Build history of the part. All positions in model axes, mm. Round coordinates to 2 decimals unless told otherwise and drop trailing zeros. Order: outer loops, then holes, each group sorted by start corner. A loop starts at its lowest first (then second) coordinate and runs counter-clockwise, first axis right, second up. Notation, with made-up numbers: M 1,53 L 52,53 A26 ccw 52,91 Z; hole C 41,51 d6. An arc over 180 degrees is marked long. One line per item, written item: value. Start each with the question number.
Item 1: Band-saw the part on A-A, the plane z = 262. Write the cut outline in (x, y).
Item 2: Band-saw the part on B-B, the plane z = 329. Write the cut outline in (x, y), then the cut area to 3 significant figures.
Item 3: Pin check, flat tips, straight feed: pin 1 (2 mm diameter, centred on y = 20, z = 311.5, fed in from -X); pin 2 (4 mm diameter, centred on y = 50.8, z = 101.6, fed in from -X); pin 3 (0.8 mm diameter, centred on x = 0.5, y = 27, fed in from -Z). Stop position of each tip, or through.
Item 4: Probe L1, parallel to Z at x = 0.4, y = 6.35; L2, parallel to Y at x = 0.55, z = 139.7; L3, parallel to Z at x = 0.1, y = -13. List the from-to ranges inside material, lowest first.
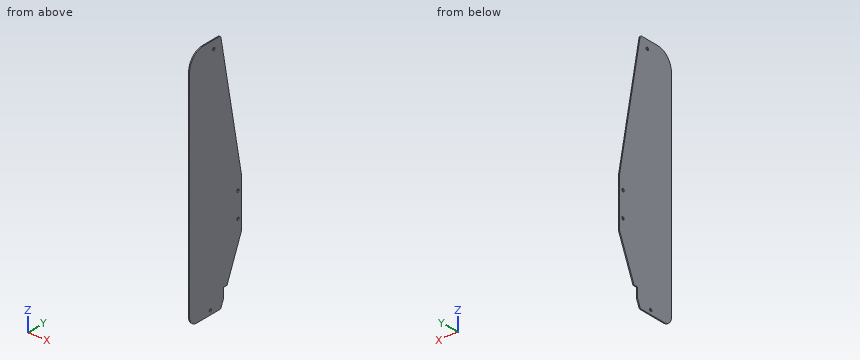
Autodesk Inventor part; units mm, degrees
ref_plane "YZ Plane" through (0, 0, 0) normal (1, 0, 0) x (0, 1, 0)
ref_plane "XZ Plane" through (0, 0, 0) normal (0, 1, 0) x (-1, 0, 0)
ref_plane "XY Plane" through (0, 0, 0) normal (0, 0, 1) x (1, 0, 0)
sketch "main" plane through (0, 0, 0) normal (0, 0, 1) x (1, 0, 0)
  circle A0 centre (51.9329, 240.4167) radius 2.1844
  line L0 (60.6642, 253.1167) -> (43.2017, 253.1167)
  arc A1 (32.8829, 253.1167) -> (7.4829, 227.7167) centre (32.8829, 227.7167) ccw
  line L1 (39.2329, 253.1167) -> (32.8829, 253.1167)
  line L2 (39.2329, 249.9417) -> (39.2329, 253.1167)
  line L3 (39.2329, 253.1167) -> (42.4079, 253.1167)
  line L4 (42.4079, 253.1167) -> (43.2017, 253.1167)
  arc A2 (65.1185, 250.5268) -> (61.9979, 253.1167) centre (61.9979, 249.9417) ccw
  line L5 (61.9979, 253.1167) -> (60.6642, 253.1167)
  line L6 (42.4079, -115.1833) -> (62.5393, -115.1833)
  arc A3 (7.4829, -102.4833) -> (20.1829, -115.1833) centre (20.1829, -102.4833) ccw
  line L7 (20.1829, -115.1833) -> (42.4079, -115.1833)
  arc A4 (62.5393, -115.1833) -> (65.4576, -113.259) centre (62.5393, -112.0083) ccw
  line L8 (39.2329, 249.9417) -> (39.2329, -115.1833)
  line L9 (102.7329, -25.6316) -> (102.7329, 49.6216)
  line L10 (102.6786, 50.2068) -> (65.1185, 250.5268)
  line L11 (7.4829, 227.7167) -> (7.4829, -102.4833)
  arc A5 (102.7329, 49.6216) -> (102.6786, 50.2068) centre (99.5579, 49.6216) ccw
  circle A6 centre (96.3829, 30.8667) radius 2.1844
  circle A7 centre (96.3829, -7.2333) radius 2.1844
  arc A8 (102.4762, -26.8823) -> (102.7329, -25.6316) centre (99.5579, -25.6316) ccw
  circle A9 centre (45.5829, -108.8333) radius 2.1844
  line L12 (65.7143, -112.66) -> (65.4576, -113.259)
  line L13 (70.0758, -102.4833) -> (70.0758, -92.9583)
  line L14 (102.4762, -26.8823) -> (76.199, -88.1958)
  line L15 (70.0758, -102.4833) -> (65.7143, -112.66)
  line L16 (70.0758, -102.4833) -> (70.0758, -89.7833)
  line L17 (70.0758, -102.4833) -> (70.0758, -88.1958)
  line L18 (70.0758, -88.1958) -> (76.199, -88.1958)
  point P0 (57.0821, 72.2396)
  point P1 (7.4829, 253.1167)
  point P2 (64.6329, -115.1833)
  point P3 (102.7329, -26.2833)
  dimension "d0" = 25.4
  dimension "d1" = 3.175
  dimension "d2" = 3.175
  dimension "d3" = 3.175
  dimension "d4" = 31.75
  dimension "d5" = 90
  dimension "d6" = 25.4
  dimension "d7" = 12.7
  dimension "d16" = 12.7
  dimension "d17" = 14.2875
sketch "Sketch1" plane through (0, 0, 0) normal (1, 0, 0) x (0, 1, 0)
  circle A0 centre (6.35, 349.25) radius 2.1844
  line L0 (15.0812, 361.95) -> (-2.3813, 361.95)
  arc A1 (-12.7, 361.95) -> (-38.1, 336.55) centre (-12.7, 336.55) ccw
  line L1 (-6.35, 361.95) -> (-12.7, 361.95)
  line L2 (-6.35, 358.775) -> (-6.35, 361.95)
  line L3 (-6.35, 361.95) -> (-3.175, 361.95)
  line L4 (-3.175, 361.95) -> (-2.3813, 361.95)
  arc A2 (19.5356, 359.3601) -> (16.415, 361.95) centre (16.415, 358.775) ccw
  line L5 (16.415, 361.95) -> (15.0812, 361.95)
  line L6 (-3.175, -6.35) -> (16.9564, -6.35)
  arc A3 (-38.1, 6.35) -> (-25.4, -6.35) centre (-25.4, 6.35) ccw
  line L7 (-25.4, -6.35) -> (-3.175, -6.35)
  arc A4 (16.9564, -6.35) -> (19.8747, -4.4257) centre (16.9564, -3.175) ccw
  line L8 (-6.35, 358.775) -> (-6.35, -6.35)
  line L9 (57.15, 83.2017) -> (57.15, 158.4549)
  line L10 (57.0956, 159.04) -> (19.5356, 359.3601)
  line L11 (-38.1, 336.55) -> (-38.1, 6.35)
  arc A5 (57.15, 158.4549) -> (57.0956, 159.04) centre (53.975, 158.4549) ccw
  circle A6 centre (50.8, 139.7) radius 2.1844
  circle A7 centre (50.8, 101.6) radius 2.1844
  arc A8 (56.8933, 81.951) -> (57.15, 83.2017) centre (53.975, 83.2017) ccw
  circle A9 centre (0, 0) radius 2.1844
  line L12 (20.1314, -3.8267) -> (19.8747, -4.4257)
  line L13 (24.4929, 6.35) -> (24.4929, 15.875)
  line L14 (56.8933, 81.951) -> (30.6161, 20.6375)
  line L15 (24.4929, 6.35) -> (20.1314, -3.8267)
  line L16 (24.4929, 6.35) -> (24.4929, 19.05)
  line L17 (24.4929, 6.35) -> (24.4929, 20.6375)
  line L18 (24.4929, 20.6375) -> (30.6161, 20.6375)
  point P0 (24.4929, 15.875)
  point P1 (24.4929, 19.05)
extrude "Extrusion1" add sketch "Sketch1" along normal blind 1.5875
feature "Bend Part1" [suppressed]
equation "\"BendRadius\" = Thickness"
equation "\"BendReliefWidth\" = Thickness"
equation "\"BendReliefDepth\" = 0.5 * Thickness"
equation "\"CornerReliefSize\" = 4 * Thickness"
equation "\"MinimumRemnant\" = 2 * Thickness"
equation "\"TransitionRadius\" = BendRadius"
equation "\"JacobiRadiusSize\" = BendRadius"
equation "\"GapSize\" = Thickness"
properties part number "side_panel" material "Acetal Resin, White"
Output:
1. outline: M 0,-38.1 L 1.59,-38.1 L 1.59,37.79 L 0,37.79 Z
2. outline: M 0,-38.1 L 1.59,-38.1 L 1.59,25.23 L 0,25.23 Z
2. area: 101 mm²
3. pin 1: stops at x = 0
3. pin 2: passes through
3. pin 3: stops at z = 20.64
4. L1: z = -6.35 to 347.07, 351.43 to 361.95
4. L2: y = -38.1 to 48.62, 52.98 to 57.15
4. L3: z = -6.35 to 361.95
